Part print with two shaded views. Sizes in mm from the minimum x, y, z corner. A direction names the side the tool comes from. Round coordinates to 2 decimals unless told otherwise and drop trailing zeros. Write each loop counter-clockwise with the first axis right and the second up, starting at its lowest first coordinate (ties: lowest second). Pieces come first, ordered by that corner, then holes. Notation, with made-up numbers: (-14.5, 34) - (1.5, 34) arc R10 ccw to (1.5, 49) - close; hole circle Ø9 at (70.25, 66.25). An arc over 180 degrees is marked (long way). Use one line per item in the form item = value. Start each with the question number.
Item 1: Pin check, flat tips, straight feed: pin 1 (6 mm diameter, centred on y = 36.5, z = 11.5, fed in from +X); pin 2 (6 mm diameter, centred on x = 17, z = 4.5, fed in from +Y); pin 3 (12 mm diameter, centred on x = 31.5, z = 21, fed in from +Y). Stop position of each tip, or through.
Item 2: Tool access for the marked faces 1 and 2: list every direction of +Z, -Z, +X, -X, +Y, -Y with a clear straight run to the whole face (end or side of a thin tool).
Item 3: Drill centre lines: L1, parallel to X at y = 17, z = 34.5; L2, parallel to X at y = 32, z = 23; L3, parallel to Y at x = 32, z = 32. Where is each one in solid material? Low to high.
Item 4: Band-saw the part on B-B, the plane y = 32. List the corners of the cut face in (x, z).
Item 5: Band-saw the part on C-C, the plane x = 23.5. List the corners of the cut face in (y, z).
Item 6: Band-saw the part on A-A, the plane z = 26.5. List the corners of the cut face in (x, y), and give its area (4 significant figures).
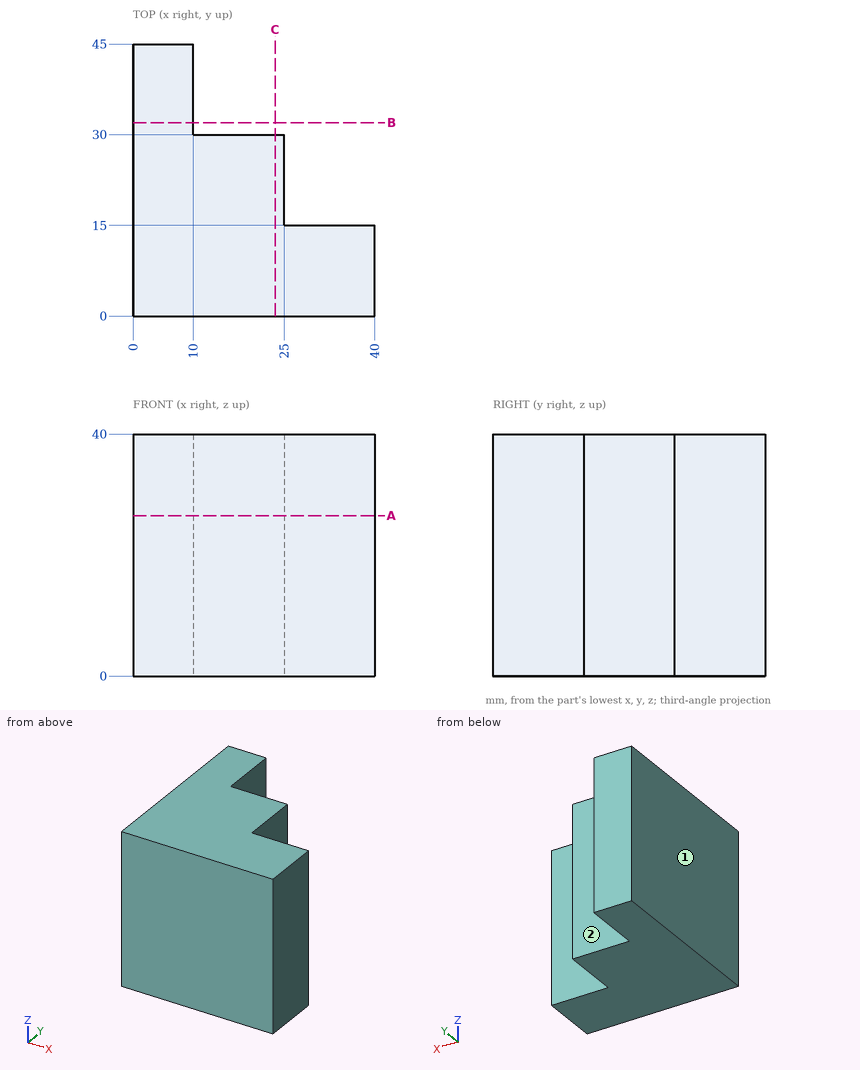
Determined:
q1.pin_1 = 10
q1.pin_2 = 30
q1.pin_3 = 15
q2.face_1 = +Z, -Z, -X, +Y, -Y
q2.face_2 = +Z, -Z, +X, +Y
q3.L1 = 0 to 25
q3.L2 = 0 to 10
q3.L3 = 0 to 15
q4.outline = (0, 0) - (10, 0) - (10, 40) - (0, 40) - close
q5.outline = (0, 0) - (30, 0) - (30, 40) - (0, 40) - close
q6.outline = (0, 0) - (40, 0) - (40, 15) - (25, 15) - (25, 30) - (10, 30) - (10, 45) - (0, 45) - close
q6.area = 1,125 mm²
